from build123d import *

# Parameters (mm, degrees)
F0_R      = 2.8
F1_DEPTH  = 1.5
F0_R_2    = 2.425
F2_DEPTH  = 2.2
F3_R      = 2.7
F4_DEPTH  = 2.5
F6_DEPTH  = 7.5
F7_R      = 3.2
F8_DEPTH  = 7
F9_R      = 1
F10_SIZE  = 0.25
F11_R     = 1.5
F12_DEPTH = 8.5


with BuildPart() as f1:
    # F0 (on Front) → F1 (new body)
    with BuildSketch(Plane.XZ):
        with BuildLine():
            Line((0, 4.8), (-3.7, 4.8))
            ThreePointArc((-3.7, 4.8), (-7.0941125497, 3.3941125497), (-8.5, 0))
            ThreePointArc((-8.5, 0), (-7.0941125497, -3.3941125497), (-3.7, -4.8))
            Line((-3.7, -4.8), (0, -4.8))
            Line((0, -4.8), (3.7, -4.8))
            ThreePointArc((3.7, -4.8), (7.0941125497, -3.3941125497), (8.5, 0))
            ThreePointArc((8.5, 0), (7.0941125497, 3.3941125497), (3.7, 4.8))
            Line((3.7, 4.8), (0, 4.8))
        make_face()
        with Locations((-3.7, 0)):
            Circle(F0_R, mode=Mode.SUBTRACT)
        with Locations((3.7, 0)):
            Circle(F0_R, mode=Mode.SUBTRACT)
    extrude(amount=-F1_DEPTH)

    # F0 (on Front) → F2 (join)
    with BuildSketch(Plane.XZ):
        with BuildLine():
            Line((0, 4.8), (-3.7, 4.8))
            ThreePointArc((-3.7, 4.8), (-7.0941125497, 3.3941125497), (-8.5, 0))
            ThreePointArc((-8.5, 0), (-7.0941125497, -3.3941125497), (-3.7, -4.8))
            Line((-3.7, -4.8), (0, -4.8))
            Line((0, -4.8), (3.7, -4.8))
            ThreePointArc((3.7, -4.8), (7.0941125497, -3.3941125497), (8.5, 0))
            ThreePointArc((8.5, 0), (7.0941125497, 3.3941125497), (3.7, 4.8))
            Line((3.7, 4.8), (0, 4.8))
        make_face()
        with Locations((-3.7, 0)):
            Circle(F0_R, mode=Mode.SUBTRACT)
        with Locations((3.7, 0)):
            Circle(F0_R, mode=Mode.SUBTRACT)
        with Locations((-3.7, 0)):
            Circle(F0_R)
        with Locations((-3.7, 0)):
            Circle(F0_R_2, mode=Mode.SUBTRACT)
        with Locations((3.7, 0)):
            Circle(F0_R)
        with Locations((3.7, 0)):
            Circle(F0_R_2, mode=Mode.SUBTRACT)
    extrude(amount=F2_DEPTH)

    # F3 (on face) → F4 (join)
    with BuildSketch(Plane.XZ.offset(2.2)):
        with BuildLine():
            ThreePointArc((3.7, -4.8), (8.5, 0), (3.7, 4.8))
            Line((3.7, 4.8), (-3.7, 4.8))
            ThreePointArc((-3.7, 4.8), (-8.5, 0), (-3.7, -4.8))
            Line((-3.7, -4.8), (3.7, -4.8))
        make_face()
        with Locations((-3.7, 0)):
            Circle(F3_R, mode=Mode.SUBTRACT)
        with Locations((3.7, 0)):
            Circle(F3_R, mode=Mode.SUBTRACT)
    extrude(amount=F4_DEPTH)

    # F5 (on face) → F6 (join)
    with BuildSketch(Plane.XZ.offset(4.7)):
        with BuildLine():
            ThreePointArc((-3.7, 4.8), (-8.5, 0), (-3.7, -4.8))
            Line((-3.7, -4.8), (3.7, -4.8))
            ThreePointArc((3.7, -4.8), (8.5, 0), (3.7, 4.8))
            Line((3.7, 4.8), (-3.7, 4.8))
        make_face()
        with BuildLine():
            Line((0, -3.8), (-3.7, -3.8))
            ThreePointArc((-3.7, -3.8), (-7.5, 0), (-3.7, 3.8))
            Line((-3.7, 3.8), (-1.7, 3.8))
            Line((-1.7, 3.8), (0, 2.1))
            Line((0, 2.1), (1.7, 3.8))
            Line((1.7, 3.8), (3.7, 3.8))
            ThreePointArc((3.7, 3.8), (7.5, 0), (3.7, -3.8))
            Line((3.7, -3.8), (0, -3.8))
        make_face(mode=Mode.SUBTRACT)
    extrude(amount=F6_DEPTH)

    # F7 (on face) → F8 (join)
    with BuildSketch(Plane(origin=(0, 1.5, 0), x_dir=(-1, 0, 0), z_dir=(0, 1, 0))):
        with BuildLine():
            ThreePointArc((3.7, -4.8), (8.5, 0), (3.7, 4.8))
            Line((3.7, 4.8), (-3.7, 4.8))
            ThreePointArc((-3.7, 4.8), (-8.5, 0), (-3.7, -4.8))
            Line((-3.7, -4.8), (3.7, -4.8))
        make_face()
        with Locations((-3.7, 0)):
            Circle(F7_R, mode=Mode.SUBTRACT)
        with Locations((3.7, 0)):
            Circle(F7_R, mode=Mode.SUBTRACT)
    extrude(amount=F8_DEPTH)

    # F9
    f9_edges = [f1.edges().sort_by_distance(p)[0] for p in [
        (0, 8.5, 4.8),
    ]]
    fillet(f9_edges, radius=F9_R)

    # F10
    f10_edges = [f1.edges().sort_by_distance(p)[0] for p in [
        (-7.5, -12.2, 0),
        (-2.7, -12.2, 3.8),
        (-0.85, -12.2, 2.95),
        (0.85, -12.2, 2.95),
        (2.7, -12.2, 3.8),
        (7.5, -12.2, 0),
        (0, -12.2, -3.8),
    ]]
    chamfer(f10_edges, length=F10_SIZE)

    # F11 (on Right) → F12 (cut, symmetric)
    with BuildSketch(Plane.YZ):
        with Locations((-2.5, 5.8)):
            Circle(F11_R)
        with Locations((1.5, 5.8)):
            Circle(F11_R)
        with Locations((5.5, 5.8)):
            Circle(F11_R)
        with Locations((-2.5, -5.8)):
            Circle(F11_R)
        with Locations((1.5, -5.8)):
            Circle(F11_R)
        with Locations((5.5, -5.8)):
            Circle(F11_R)
    extrude(amount=F12_DEPTH, both=True, mode=Mode.SUBTRACT)


solid = f1.part
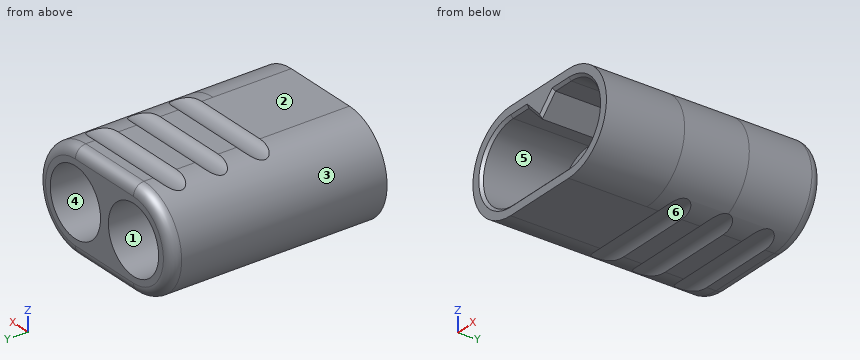
Design review of the part built by this model. Coordinates are the model's own, in mm. Face numbers are marked on the shaded views. A direction names the side the tool comes from. Coordinates: 2 decimals unless noted, no trailing zeros. Order: outer loops, then holes, each group sorted by start corner. A loop starts at its lowest first (then second) coordinate and runs counter-clockwise, first axis right, second up.
Item 1: For the marked faces 4, 5 and 6, list the 3-axis set-ups (+Z, -Z, +X, -X, +Y, -Y) from which the entire face can be reached by the end or side of a thin tool; tool diameter is ignored.
Item 2: Take a section at A-A, the plane y = 7. Write out the cut boundary in (x, z), then the cut area to 3 significant figures.
Item 3: For pin 1 Ø2.5 at (x, z) = (-2, 1) entering from -Y; pin 2 Ø5 at (y, z) = (-2, -3) entering from +X; pin 3 Ø1.7 at (x, z) = (-4.5, 0) entering from +Y; pin 4 Ø5 at (x, z) = (3.7, 0) entering from +Y, all flat-tipped, find the tip position at first contact; note any pin that passes through.
Item 4: For line 1 (Z direction, x = 3.7, y = -3.8); line 2 (X direction, y = -7.5, z = 3); line 3 (Z direction, x = 3.7, y = -0.95) (3 decimals), list the stretches that pass through material, from the lowest coordinate up.
Item 5: The part is to be moulded in two halves that separate along Z. For the marked faces 1, 2 and 3, say which applies: pulls with the +Z half, pulls with the -Z half, needs draft (parallel to the pull), parting line crosses it, or undercut.
The answers:
1. face 4: +Y
1. face 5: -Y
1. face 6: -Z, +X, -X
2. outline: (-3.7, -4.8) - (3.7, -4.8) arc R4.8 ccw to (3.7, 4.8) - (-3.7, 4.8) arc R4.8 ccw to start; hole circle Ø6.4 at (-3.7, 0); hole circle Ø6.4 at (3.7, 0)
2. area: 79.1 mm2
3. pin 1: stops at y = -4.7
3. pin 2: stops at x = 8.47
3. pin 3: passes through
3. pin 4: stops at y = 0
4. line 1: z = -4.8 to -2.7, 2.7 to 4.8
4. line 2: x = -7.45 to -6.03, -0.9 to 0.9, 6.03 to 7.45
4. line 3: z = -4.8 to -2.425, 2.425 to 4.8
5. face 1: undercut
5. face 2: pulls with the +Z half
5. face 3: parting line crosses it
